Part model, mm, in its own coordinate system. A direction names the side the tool comes from. Round coordinates to 2 decimals unless told otherwise and drop trailing zeros. Write each loop counter-clockwise with the first axis right and the second up, starting at its lowest first coordinate (ties: lowest second). Pieces come first, ordered by that corner, then holes.
```python
from build123d import *

# Parameters (mm, degrees)
BOSS_EXTRUDE1_DEPTH = 558.8


with BuildPart() as part:
    # Sketch1 → Boss-Extrude1 (new body)
    with BuildSketch(Plane(origin=(0, 0, 0), x_dir=(0, 0, -1), z_dir=(1, 0, 0))):
        with BuildLine():
            Line((0, 16.231012583), (0, -315.218136756))
            Line((0, -315.218136756), (-112.188138154, -315.218136756))
            Line((-112.188138154, -315.218136756), (-161.738988814, -364.768987417))
            Line((-161.738988814, -364.768987417), (0, -364.768987417))
            Line((0, -364.768987417), (9.710862229, -364.768987417))
            Line((9.710862229, -364.768987417), (9.710862229, 16.231012583))
            ThreePointArc((9.710862229, 16.231012583), (-2.234969693, 45.070802024), (-31.074759134, 57.016633947))
            Line((-31.074759134, 57.016633947), (-112.188138154, 31.76839215))
            Line((-112.188138154, 31.76839215), (-112.188138154, 16.231012583))
            Line((-112.188138154, 16.231012583), (-31.074759134, 47.305771717))
            ThreePointArc((-31.074759134, 47.305771717), (-9.101586227, 38.204185491), (0, 16.231012583))
        make_face()
    extrude(amount=BOSS_EXTRUDE1_DEPTH)


solid = part.part
```
Q1. Wall check: L1, parallel to Z at x = 56, y = -225; L2, parallel to Y at x = 140.5, z = 92.5; L3, parallel to Y at x = 456.5, z = 61. Give the ranges that are in metal, low to high.
Values follow:
L1: z = -9.71 to 0
L2: y = -364.77 to -315.22, 23.77 to 37.9
L3: y = -364.77 to -315.22, 35.84 to 47.7
Q2. Which spindle directions (+Z, -Z, +X, -X, +Y, -Y) get a long thin tool onto all of the face, cutting with end or side? Do faces 4 (the flat face through (275, 24, 112.188)), 5 (the flat face through (275, -315.218, 55)), 6 (the flat face through (275, -177, -9.711)), 7 (the cylindrical face through (275.5, 38.4, 9.3)). Say none if no direction does.
Values follow:
face 4: +Z, +X, -X, +Y
face 5: +Z, +X, -X
face 6: -Z, +X, -X, +Y, -Y
face 7: +X, -X
Q3. Cut at B-B on x = 419.5. Write the cut outline in (y, z), plus the area to 3 significant figures.
Values follow:
outline: (-364.77, -9.71) - (16.23, -9.71) arc R40.79 ccw to (57.02, 31.07) - (31.77, 112.19) - (16.23, 112.19) - (47.31, 31.07) arc R31.07 cw to (16.23, 0) - (-315.22, 0) - (-315.22, 112.19) - (-364.77, 161.74) - close
area: 12,100 mm2
Q4. Cut at C-C on y = -136. Write the cut outline in (x, z).
Values follow:
outline: (0, -9.71) - (558.8, -9.71) - (558.8, 0) - (0, 0) - close
Q5. Cut at A-A on z = 55. Write the cut outline in (x, y).
Values follow:
outline: (0, -364.77) - (558.8, -364.77) - (558.8, -315.22) - (0, -315.22) - close; (0, 38.14) - (558.8, 38.14) - (558.8, 49.57) - (0, 49.57) - close
Q6. Cut at D-D on z = 100.5. Write the cut outline in (x, y).
Values follow:
outline: (0, -364.77) - (558.8, -364.77) - (558.8, -315.22) - (0, -315.22) - close; (0, 20.71) - (558.8, 20.71) - (558.8, 35.41) - (0, 35.41) - close
Q7. Mould opens along Y. For faces 1 (the flat face through (275, -364.769, 77)), 2 (the flat face through (275.49, -339.65, 136.62)), 3 (the flat face through (275, -147, 0)) say: +Y half, -Y half, draft (parallel to the pull), parting line (faces both ways), or undercut.
Values follow:
face 1: -Y half
face 2: +Y half
face 3: undercut
Q8. Drop flat-ended pins along their axis: pin 1 (4.5 mm diameter, centred on x = 354.5, y = 27, fed in from +Z); pin 2 (6 mm diameter, centred on x = 475.5, z = 87, fed in from +Y); pin 3 (6 mm diameter, centred on x = 407, y = -243.5, fed in from +Z). Give the stop position or say it passes through.
Values follow:
pin 1: stops at z = 112.19
pin 2: stops at y = 40.54
pin 3: stops at z = 0
